Work out the finished part from the listing and answer in its coordinate system (mm). A direction names the side the tool comes from. Round coordinates to 2 decimals unless told otherwise and drop trailing zeros. Loops run counter-clockwise (first coordinate to the right, second up) from the corner with the lowest first, then second, coordinate; pieces in that order, holes last.
```python
from build123d import *

# Parameters (mm, degrees)
SKETCH1_W           = 225
SKETCH1_H           = 55
BOSS_EXTRUDE1_DEPTH = 54
SHELL1_T            = -4
SKETCH2_R           = 2
CUT_EXTRUDE1_DEPTH  = 10


with BuildPart() as part:
    # Sketch1 → Boss-Extrude1 (new body)
    with BuildSketch(Plane.XY):
        with Locations((112.5, -27.5)):
            Rectangle(SKETCH1_W, SKETCH1_H)
    extrude(amount=BOSS_EXTRUDE1_DEPTH)

    # Shell1
    shell1_openings = [part.faces().sort_by_distance(p)[0] for p in [
        (0, -27.5, 27),
    ]]
    offset(amount=SHELL1_T, openings=shell1_openings, kind=Kind.INTERSECTION)

    # Sketch2 → Cut-Extrude1 (cut)
    with BuildSketch(Plane(origin=(0, 0, 0), x_dir=(1, 0, 0), z_dir=(0, 1, 0))):
        with Locations((12.5, -12.998097245)):
            Circle(SKETCH2_R)
        with Locations((212.5, -12.998097245)):
            Circle(SKETCH2_R)
        with Locations((212.5, -41.001902755)):
            Circle(SKETCH2_R)
        with Locations((12.5, -41.001902755)):
            Circle(SKETCH2_R)
    extrude(amount=-CUT_EXTRUDE1_DEPTH, mode=Mode.SUBTRACT)


solid = part.part
```
1. Find section B-B (z = 18). Write down the section's boundary in (x, y), then the cut area to 3 significant figures.
Answer key:
outline: (0, -55) - (225, -55) - (225, 0) - (0, 0) - (0, -4) - (221, -4) - (221, -51) - (0, -51) - close
area: 1,990 mm2
2. Given pin 1 (5 mm diameter, centred on x = 100, z = 19.5, fed in from +Y); pin 2 (2.5 mm diameter, centred on x = 212.5, z = 41, fed in from +Y); pin 3 (14 mm diameter, centred on y = -35, z = 26.5, fed in from -X), each flat-ended and moving along its own axis, determine where each tip first touches the part or whether it passes through.
Answer key:
pin 1: stops at y = 0
pin 2: stops at y = -51
pin 3: stops at x = 221
3. Consider probe 1 along Z at (x, y) = (212.5, -2.65); probe 2 along Y at (x, z) = (170, 31); probe 3 along Z at (x, y) = (195, -14.5). Determine where each line is inside the solid, lowest interval first.
Answer key:
probe 1: z = 0 to 11, 15 to 39, 43 to 54
probe 2: y = -55 to -51, -4 to 0
probe 3: z = 0 to 4, 50 to 54
4. Find section C-C (x = 159.5). Write down the section's boundary in (y, z), then the cut area to 3 significant figures.
Answer key:
outline: (-55, 0) - (0, 0) - (0, 54) - (-55, 54) - close; hole (-51, 4) - (-4, 4) - (-4, 50) - (-51, 50) - close
area: 808 mm2
5. Find section D-D (y = -11). Write down the section's boundary in (x, z).
Answer key:
outline: (0, 0) - (225, 0) - (225, 54) - (0, 54) - (0, 50) - (221, 50) - (221, 4) - (0, 4) - close
6. Determine the mould class of faces 1 (the face through (225, -28, 27)), 2 (the face through (111, 0, 27)), 3 (the face through (221, -28, 27)) for opening direction Y: +Y half, -Y half, draft (parallel to the pull), parting line (faces both ways), or undercut.
Answer key:
face 1: draft
face 2: +Y half
face 3: undercut
7. Which of the six approach directions +Z, -Z, +X, -X, +Y, -Y give full straight-line access (tool end or side, diameter ignored) to faces 4 (the face through (11.026, -1.972, 39.65)), 5 (the face through (111, -27, 0)), 6 (the face through (109, -51, 27))?
Answer key:
face 4: +Y
face 5: -Z, +X, -X, +Y, -Y
face 6: -X
8. Find section A-A (x = 12.5). Write down the section's boundary in (y, z), then the cut area to 3 significant figures.
Answer key:
outline: (-55, 0) - (0, 0) - (0, 11) - (-4, 11) - (-4, 4) - (-51, 4) - (-51, 50) - (-4, 50) - (-4, 43) - (0, 43) - (0, 54) - (-55, 54) - close; (-4, 15) - (0, 15) - (0, 39) - (-4, 39) - close
area: 776 mm2
